Geometry: final body of the model. Coordinates: model frame, mm. Face numbers are marked on the shaded views. A direction names the side the tool comes from. Give positions to 0.01 mm unless a question says otherwise; leave off trailing zeros. Order: outer loops, then holes, each group sorted by start corner. A loop starts at its lowest first (then second) coordinate and runs counter-clockwise, first axis right, second up. Notation, with made-up numbers: (-9.5, 41.5) -> (47.5, 41.5) arc R8 ccw to (47.5, 45.5) -> close; hole circle Ø4 at (57.5, 59). An arc over 180 degrees is marked (long way). Answer in a Markdown table with one row per item. Add a question column.
Q1. Line query: line 1 along Z through (x, y) = (-30, 16); line 2 along X through (y, z) = (16, 5); line 3 along Y through (x, z) = (14, 11.75). Output: solid intervals per line, ascending. Write a range as from..to.
Q2. Cut plane B-B on y = -7. Return the cut outline in (x, z).
Q3. Set-up query: the marked faces 5, 6 and 7. Return all of +Z, -Z, +X, -X, +Y, -Y with unobstructed straight access to the full face (end or side cutting, diameter ignored); none if empty.
Q4. Contact query for flat-ended pins moving along their axis: P1, Ø11.5, axis at x = 14.5, y = -12, coming from the +Z side; P2, Ø3, axis at x = -30, z = 15, coming from the -Y side; P3, Ø1.4, axis at y = -10.5, z = 18, coming from the -X side; P4, Ø2, axis at x = 30, z = 15, coming from the -Y side. Output: stop coordinate, or through.
Q5. Cut plane A-A on z = 11.75. Return the cut outline in (x, y).
Q6. Pull-direction query (Y, two-part tool) for the marked faces 1, 2, 3 and 4; classes: +Y half, -Y half, draft (parallel to the pull), parting line (faces both ways), or undercut.
Q7. Cut plane C-C on z = 18.25. Return the cut outline in (x, y).
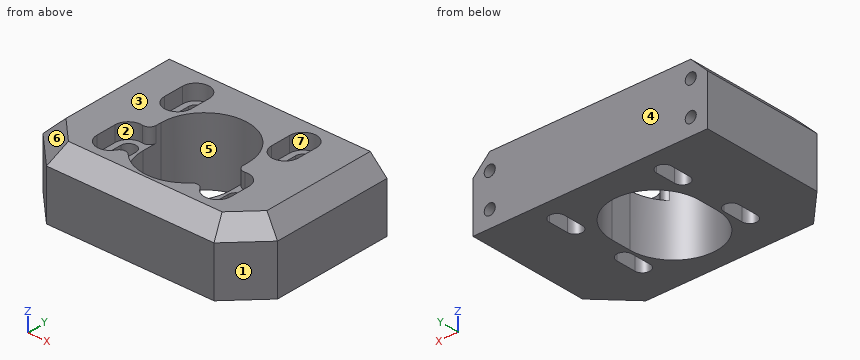
from build123d import *

# Parameters (mm, degrees)
SKETCH1_W                                            = 70
SKETCH1_H                                            = 46.5
BOSS_EXTRUDE1_DEPTH                                  = 20
CUT_EXTRUDE1_DEPTH                                   = 47.535604648
CBORE_FOR_M4_HEXAGON_SOCKET_HEAD_CAP_SCR_D           = 4.5
CBORE_FOR_M4_HEXAGON_SOCKET_HEAD_CAP_SCR_CBORE_D     = 8
CBORE_FOR_M4_HEXAGON_SOCKET_HEAD_CAP_SCR_CBORE_DEPTH = 4.6
CUT_EXTRUDE2_DEPTH                                   = 45.751787674
CUT_EXTRUDE3_DEPTH                                   = 45.751787674
FILLET1_R                                            = 2
CHAMFER1_SIZE                                        = 10
M4_TAPPED_HOLE1_D                                    = 3.3
M4_TAPPED_HOLE1_DEPTH                                = 10
M4_TAPPED_HOLE1_TIP                                  = 0.991420021
CHAMFER2_SIZE                                        = 5


with BuildPart() as part:
    # Sketch1 → Boss-Extrude1 (new body)
    with BuildSketch(Plane.XY):
        Rectangle(SKETCH1_W, SKETCH1_H)
    extrude(amount=BOSS_EXTRUDE1_DEPTH)

    # Sketch2 → Cut-Extrude1 (cut, through all)
    with BuildSketch(Plane.XY.offset(20)):
        with BuildLine():
            Line((-13, -4.5), (-13, 1.5))
            ThreePointArc((-13, 1.5), (0, 14.5), (13, 1.5))
            Line((13, 1.5), (13, -4.5))
            ThreePointArc((13, -4.5), (0, -17.5), (-13, -4.5))
        make_face()
    extrude(amount=-CUT_EXTRUDE1_DEPTH, mode=Mode.SUBTRACT)

    # CBORE for M4 Hexagon socket head cap screws1 (through all)
    with Locations(Plane.XY.offset(20)):
        with Locations((-16, 13.5), (-16, -9), (16, -9), (16, 13.5), (0, -1.5)):
            CounterBoreHole(CBORE_FOR_M4_HEXAGON_SOCKET_HEAD_CAP_SCR_D / 2, CBORE_FOR_M4_HEXAGON_SOCKET_HEAD_CAP_SCR_CBORE_D / 2, CBORE_FOR_M4_HEXAGON_SOCKET_HEAD_CAP_SCR_CBORE_DEPTH)

    # Sketch6 → Cut-Extrude2 (cut, through all)
    with BuildSketch(Plane.XY.offset(15.4)):
        with BuildLine():
            Line((-12, 16.5), (-12, 10.5))
            ThreePointArc((-12, 10.5), (-16, 6.5), (-20, 10.5))
            Line((-20, 10.5), (-20, 16.5))
            ThreePointArc((-20, 16.5), (-16, 20.5), (-12, 16.5))
        make_face()
        with BuildLine():
            Line((-12, -6), (-12, -12))
            ThreePointArc((-12, -12), (-16, -16), (-20, -12))
            Line((-20, -12), (-20, -6))
            ThreePointArc((-20, -6), (-16, -2), (-12, -6))
        make_face()
        with BuildLine():
            Line((20, 16.5), (20, 10.5))
            ThreePointArc((20, 10.5), (16, 6.5), (12, 10.5))
            Line((12, 10.5), (12, 16.5))
            ThreePointArc((12, 16.5), (16, 20.5), (20, 16.5))
        make_face()
        with BuildLine():
            Line((12, -12), (12, -6))
            ThreePointArc((12, -6), (16, -2), (20, -6))
            Line((20, -6), (20, -12))
            ThreePointArc((20, -12), (16, -16), (12, -12))
        make_face()
    extrude(amount=CUT_EXTRUDE2_DEPTH, mode=Mode.SUBTRACT)

    # Sketch7 → Cut-Extrude3 (cut, through all)
    with BuildSketch(Plane.XY.offset(15.4)):
        with BuildLine():
            Line((-13.75, 16.5), (-13.75, 10.5))
            ThreePointArc((-13.75, 10.5), (-16, 8.25), (-18.25, 10.5))
            Line((-18.25, 10.5), (-18.25, 16.5))
            ThreePointArc((-18.25, 16.5), (-16, 18.75), (-13.75, 16.5))
        make_face()
        with BuildLine():
            Line((-18.25, -12), (-18.25, -6))
            ThreePointArc((-18.25, -6), (-16, -3.75), (-13.75, -6))
            Line((-13.75, -6), (-13.75, -12))
            ThreePointArc((-13.75, -12), (-16, -14.25), (-18.25, -12))
        make_face()
        with BuildLine():
            Line((18.25, 16.5), (18.25, 10.5))
            ThreePointArc((18.25, 10.5), (16, 8.25), (13.75, 10.5))
            Line((13.75, 10.5), (13.75, 16.5))
            ThreePointArc((13.75, 16.5), (16, 18.75), (18.25, 16.5))
        make_face()
        with BuildLine():
            Line((18.25, -6), (18.25, -12))
            ThreePointArc((18.25, -12), (16, -14.25), (13.75, -12))
            Line((13.75, -12), (13.75, -6))
            ThreePointArc((13.75, -6), (16, -3.75), (18.25, -6))
        make_face()
    extrude(amount=-CUT_EXTRUDE3_DEPTH, mode=Mode.SUBTRACT)

    # Fillet1
    # the kernel refuses this fillet: 2 mm, written as the material it takes off along each edge
    with BuildSketch(Plane(origin=(13, -3.354248689, 28.17582118), x_dir=(0.8738382268582209, 0.48621677601794083, 0), z_dir=(0, 0, -1))) as fillet1_piece_1:
        with BuildLine():
            CenterArc((3.33776502, -1.885304481), FILLET1_R, 109.498154832, 99.594068227)
            Line((1.590088566, -2.857738033), (0, 0))
            ThreePointArc((0, 0), (1.335106008, -0.229391038), (2.670212016, 0))
        make_face()
    extrude(amount=12.77582118, mode=Mode.SUBTRACT)
    with BuildSketch(Plane(origin=(12, -9.5, 15.4), x_dir=(0.11433437649297556, -0.993442323616204, 0), z_dir=(0, 0, 1))) as fillet1_piece_2:
        with BuildLine():
            CenterArc((5.264320611, -1.843966677), FILLET1_R, 112.782223337, 106.542245194)
            Line((3.717181311, -3.111389253), (3.562467381, -3.238131511))
            ThreePointArc((3.562467381, -3.238131511), (1.876525646, -1.534267667), (-0.097526525, -0.174609785))
            Line((-0.097526525, -0.174609785), (0.022866875, 0.198688465))
            ThreePointArc((0.022866875, 0.198688465), (2.506472684, -0.087147477), (4.412415603, 0.184396668))
            Line((4.412415603, 0.184396668), (4.489861512, 0))
        make_face()
    extrude(amount=16.718730334, mode=Mode.SUBTRACT)
    with BuildSketch(Plane(origin=(-12, -9.5, 15.4), x_dir=(0.549971838681665, -0.8351831994581241, 0), z_dir=(0, 0, 1))) as fillet1_piece_3:
        with BuildLine():
            CenterArc((5.220376144, -1.964931936), FILLET1_R, 100.745216059, 106.542245194)
            Line((3.442940977, -2.881842089), (3.265197461, -2.973533104))
            ThreePointArc((3.265197461, -2.973533104), (1.977963631, -1.541966237), (-0.109994368, -0.16703664))
            Line((-0.109994368, -0.16703664), (0.037288401, 0.196493194))
            ThreePointArc((0.037288401, 0.196493194), (2.423746067, -0.027942413), (4.810203733, 0.196493194))
            Line((4.810203733, 0.196493194), (4.847492134, 0))
        make_face()
    extrude(amount=16.718730334, mode=Mode.SUBTRACT)
    with BuildSketch(Plane(origin=(-13, -3.354248689, 28.17582118), x_dir=(-0.8738382268582207, 0.48621677601794133, 0), z_dir=(0, 0, -1))) as fillet1_piece_4:
        with BuildLine():
            CenterArc((3.33776502, 1.885304481), FILLET1_R, 150.907776941, 99.594068227)
            Line((1.590088566, 2.857738033), (0, 0))
            ThreePointArc((0, 0), (1.335106008, 0.229391038), (2.670212016, 0))
        make_face()
    extrude(amount=12.77582118, mode=Mode.SUBTRACT)

    # Chamfer1
    chamfer1_edges = [part.edges().sort_by_distance(p)[0] for p in [
        (35, -23.25, 10),
        (-35, -23.25, 10),
    ]]
    chamfer(chamfer1_edges, length=CHAMFER1_SIZE)

    # M4 Tapped Hole1
    with Locations(Plane(origin=(0, 23.25, 0), x_dir=(1, 0, 0), z_dir=(0, 1, 0))):
        with Locations((-30, -15), (-30, -5), (30, -5), (30, -15)):
            Hole(M4_TAPPED_HOLE1_D / 2, depth=M4_TAPPED_HOLE1_DEPTH)
            with Locations((0, 0, -(M4_TAPPED_HOLE1_DEPTH + M4_TAPPED_HOLE1_TIP / 2))):  # 118° drill point
                Cone(0, M4_TAPPED_HOLE1_D / 2, M4_TAPPED_HOLE1_TIP, mode=Mode.SUBTRACT)

    # Chamfer2
    chamfer2_edges = [part.edges().sort_by_distance(p)[0] for p in [
        (35, 5, 20),
        (0, -23.25, 20),
        (-30, -18.25, 20),
        (30, -18.25, 20),
        (-35, 5, 20),
    ]]
    chamfer(chamfer2_edges, length=CHAMFER2_SIZE)


solid = part.part
Completed:
| question | item | result |
|---|---|---|
| 1 | line 1 | z = 0..3.35, 6.65..13.35, 16.65..20 |
| 1 | line 2 | x = -35..-31.65, -28.35..-18.25, -13.75..13.75, 18.25..28.35, 31.65..35 |
| 1 | line 3 | y = -23.25..-13.03, -4.97..9.47, 17.53..23.25 |
| 2 | outline | (-35, 0) -> (-18.25, 0) -> (-18.25, 15.4) -> (-20, 15.4) -> (-20, 20) -> (-30, 20) -> (-35, 15) -> close; (-13.75, 0) -> (-12.76, 0) -> (-12.76, 15.4) -> (-13.75, 15.4) -> close; (12.76, 0) -> (13.75, 0) -> (13.75, 15.4) -> (12.76, 15.4) -> close; (18.25, 0) -> (35, 0) -> (35, 15) -> (30, 20) -> (20, 20) -> (20, 15.4) -> (18.25, 15.4) -> close |
| 3 | face 5 | +Z, -Z |
| 3 | face 6 | +Z, -X, -Y |
| 3 | face 7 | +Z |
| 4 | P1 | stops at z = 20 |
| 4 | P2 | stops at y = -19.75 |
| 4 | P3 | stops at x = -32.7 |
| 4 | P4 | stops at y = -19.25 |
| 5 | outline | (-35, -13.25) -> (-25, -23.25) -> (25, -23.25) -> (35, -13.25) -> (35, 23.25) -> (-35, 23.25) -> close; hole (-18.25, -12) arc R2.25 ccw to (-13.75, -12) -> (-13.75, -6) arc R2.25 ccw to (-18.25, -6) -> close; hole (-18.25, 10.5) arc R2.25 ccw to (-13.75, 10.5) -> (-13.75, 16.5) arc R2.25 ccw to (-18.25, 16.5) -> close; hole (-13, -4.5) arc R13 ccw to (13, -4.5) -> (13, 1.5) arc R13 ccw to (-13, 1.5) -> close; hole (13.75, -12) arc R2.25 ccw to (18.25, -12) -> (18.25, -6) arc R2.25 ccw to (13.75, -6) -> close; hole (13.75, 10.5) arc R2.25 ccw to (18.25, 10.5) -> (18.25, 16.5) arc R2.25 ccw to (13.75, 16.5) -> close |
| 6 | face 1 | -Y half |
| 6 | face 2 | undercut |
| 6 | face 3 | draft |
| 6 | face 4 | +Y half |
| 7 | outline | (-31.75, -11.9) -> (-23.65, -20) -> (23.65, -20) -> (31.75, -11.9) -> (31.75, 23.25) -> (-31.75, 23.25) -> close; hole (-20, -12) arc R4 ccw to (-12.51, -13.96) arc R2 cw to (-9.33, -13.55) arc R13 ccw to (9.33, -13.55) arc R2 cw to (12.51, -13.96) arc R4 ccw to (20, -12) -> (20, -6) arc R4 ccw to (15.33, -2.06) arc R2 cw to (13, -0.08) -> (13, 1.5) arc R13 ccw to (-13, 1.5) -> (-13, -0.08) arc R2 cw to (-15.33, -2.06) arc R4 ccw to (-20, -6) -> close; hole (-20, 10.5) arc R4 ccw to (-12, 10.5) -> (-12, 16.5) arc R4 ccw to (-20, 16.5) -> close; hole (12, 10.5) arc R4 ccw to (20, 10.5) -> (20, 16.5) arc R4 ccw to (12, 16.5) -> close |
